Autodesk Inventor part; units mm, degrees
ref_plane "YZ Plane" through (0, 0, 0) normal (1, 0, 0) x (0, 1, 0)
ref_plane "XZ Plane" through (0, 0, 0) normal (0, 1, 0) x (-1, 0, 0)
ref_plane "XY Plane" through (0, 0, 0) normal (0, 0, 1) x (1, 0, 0)
sketch "Sketch1" plane through (0, 0, 0) normal (0, 1, 0) x (-1, 0, 0)
  line L0 (6.6946, 16.8791) -> (-27.3054, 16.8791)
  line L1 (-32.3054, 11.8791) -> (-32.3054, -32.1209)
  line L2 (-27.3054, -37.1209) -> (6.6946, -37.1209)
  line L3 (6.6946, -37.1209) -> (6.6946, 16.8791)
  arc A0 (-27.3054, 16.8791) -> (-32.3054, 11.8791) centre (-27.3054, 11.8791) ccw
  arc A1 (-32.3054, -32.1209) -> (-27.3054, -37.1209) centre (-27.3054, -32.1209) ccw
  circle A2 centre (-22.3054, 7.8791) radius 5
  circle A3 centre (-22.3054, -28.1209) radius 5
  point P0 (0, 0)
  point P1 (-32.3054, -37.1209)
  point P2 (-32.3054, 16.8791)
  dimension "d0" = 39
  dimension "d1" = 54
  dimension "d2" = 5
  dimension "d3" = 5
  dimension "d5" = 10
  dimension "d6" = 10
  dimension "d7" = 9
  dimension "d8" = 9
extrude "Extrusion1" add sketch "Sketch1" along normal blind 8
sketch "Sketch2" plane through (0, 0, 0) normal (0, -1, 0) x (1, 0, 0)
  line L0 (-6.6946, -37.1209) -> (-6.6946, 16.8791)
  line L1 (-6.6946, 16.8791) -> (1.3054, 16.8791)
  line L2 (-6.6946, 16.8791) -> (27.3054, 16.8791)
  line L3 (1.3054, 16.8791) -> (1.3054, -37.1209)
  line L4 (27.3054, -37.1209) -> (-6.6946, -37.1209)
  line L5 (-6.6946, -37.1209) -> (1.3054, -37.1209)
  line L6 (-6.6946, -37.1209) -> (-6.6946, 16.8791)
  point P0 (0, 0)
  dimension "d11" = 8
extrude "Extrusion2" cut sketch "Sketch2" against normal blind 4
ref_plane "Work Plane1" through (1.3054, 0, -37.1209) normal (-1, 0, 0) x (0, 0, 1)
sketch "Sketch3" plane through (1.3054, 0, -37.1209) normal (-1, 0, 0) x (0, 0, 1)
  line L0 (54, 0) -> (54, 8)
  circle A0 centre (27, -44) radius 5
  arc A1 (15, -44) -> (39, -44) centre (27, -44) ccw
  line L1 (39, -44) -> (39, 0)
  line L2 (49, 0) -> (5, 0)
  line L3 (15, -44) -> (15, 0)
  line L4 (39, 0) -> (15, 0)
  point P0 (37.1209, 0)
  dimension "d17" = 10
  dimension "d18" = 24
extrude "Extrusion3" add sketch "Sketch3" against normal blind 8
sketch "Sketch4" plane through (1.3054, 0, 16.8791) normal (-1, 0, 0) x (0, 0, 1)
  line L0 (0, 4) -> (0, 0)
  circle A0 centre (-27, -44) radius 12
  point P0 (-16.8791, 0)
  dimension "d23" = 24
extrude "Extrusion4" add sketch "Sketch4" along normal blind 8
sketch "Sketch5" plane through (-6.6946, -44, -10.1209) normal (-1, 0, 0) x (0, 0, 1)
  circle A0 centre (0, 0) radius 5
  point P0 (10.1209, 44)
  dimension "d26" = 10
extrude "Extrusion5" cut sketch "Sketch5" against normal blind 8
fillet "Face Fillet1" radius 5 1 edges at (5.3054, 0, 1.8791)
fillet "Face Fillet2" radius 5 1 edges at (5.3054, 0, -22.1209)
properties part number "yatak"
The model under review builds one solid part; all positions refer to its coordinate system, in mm. A direction names the side the tool comes from. Round coordinates to 2 decimals unless told otherwise and drop trailing zeros. Loops run counter-clockwise (first coordinate to the right, second up) from the corner with the lowest first, then second, coordinate; pieces in that order, holes last. Notation, with made-up numbers: (-18, 63.25) -> (-3, 63.25) arc R15 cw to (-3, 73.25) -> close; hole circle Ø9 at (87, 83.25). An arc over 180 degrees is marked (long way). One line per question, with ' | ' between items. Start each with the question number.
Item 1: Add section A-A, the plane x = 0. Write out the cut boundary in (y, z), then the cut area to 3 significant figures.
Item 2: Add section D-D, the plane y = -18.5. Write out the cut boundary in (x, z), then the cut area to 3 significant figures.
Item 3: Add section B-B, the plane z = 10. Write out the cut boundary in (x, y), then the cut area to 3 significant figures.
Item 4: Draft analysis for pull direction Y (two halves, no side actions). For faces 1 (the face through (-0.36, -55.9, -11.68)), 2 (the face through (30.802, 3.944, -35.695)), 3 (the face through (5.361, -1.504, 3.305)), state which applies: +Y half, -Y half, draft (parallel to the pull), parting line (faces both ways), or undercut.
Item 5: Add section C-C, the plane y = -42. Write out the cut boundary in (x, z).
Item 6: Machinability: for faces 4 (the face through (9.305, -28, -10)), 5 (the face through (5, -25, 1.879)), 6 (the face through (-3, 4, -10)), which of the approach directions +Z, -Z, +X, -X, +Y, -Y give a long, thin tool a straight path to every point of the face, cutting with its end or side? Answer none if there is none.
Item 7: For pin 1 (2 mm diameter, centred on x = 4, y = -11.5, fed in from -Z); pin 2 (11.5 mm diameter, centred on x = 22.31, z = 7.88, fed in from -Y); pin 3 (12 mm diameter, centred on x = 12, y = -26.5, fed in from +Z); pin 4 (12 mm diameter, centred on y = -2, z = -24.5, fed in from +X), all flat-tipped, find the tip position at first contact; note any pin that passes through.
Item 8: Wall thickness on line 1 along Y through (x, z) = (0, -12); line 2 along Y through (x, z) = (28, -3); line 3 along X through (y, z) = (-22.5, -18.5): over which ranges is each line inside the solid? List them lowest first. Write a range as [from, to].
Return value:
1) outline: circle Ø24 at (-44, -10.12); (4, -37.12) -> (8, -37.12) -> (8, 16.88) -> (4, 16.88) -> close; hole circle Ø10 at (-44, -10.12) | area: 590 mm2
2) outline: (1.31, -22.12) -> (9.31, -22.12) -> (9.31, 1.88) -> (1.31, 1.88) -> close | area: 192 mm2
3) outline: (-6.69, 4) -> (1.31, 4) -> (1.31, 0) -> (17.78, 0) -> (17.78, 8) -> (-6.69, 8) -> close; (26.83, 0) -> (32.31, 0) -> (32.31, 8) -> (26.83, 8) -> close | area: 208 mm2
4) face 1: undercut | face 2: draft | face 3: -Y half
5) outline: (-6.69, -21.95) -> (1.31, -21.95) -> (1.31, -22.12) -> (9.31, -22.12) -> (9.31, -14.7) -> (-6.69, -14.7) -> close; (-6.69, -5.54) -> (9.31, -5.54) -> (9.31, 1.88) -> (1.31, 1.88) -> (1.31, 1.71) -> (-6.69, 1.71) -> close
6) face 4: +Z, -Z, +X, -Y | face 5: +Z, +X, -X, -Y | face 6: +Z, -Z, -X
7) pin 1: stops at z = -22.12 | pin 2: stops at y = 0 | pin 3: stops at z = 1.88 | pin 4: stops at x = 32.31
8) line 1: y = [-55.85, -48.63], [-39.37, -32.15], [4, 8] | line 2: y = [0, 8] | line 3: x = [1.31, 9.31]
